Geometry check sheet. Reference: the model listing, model coordinates, mm. A direction names the side the tool comes from. Round coordinates to 2 decimals unless told otherwise and drop trailing zeros. Order: outer loops, then holes, each group sorted by start corner. A loop starts at its lowest first (then second) coordinate and runs counter-clockwise, first axis right, second up.
(1) Gauge pin test, flat ends, axial feed: P1, Ø1, axis at x = 761.5, y = 280.5, coming from the +Z side; P2, Ø12, axis at x = 488.5, y = 11.5, coming from the +Z side; P3, Ø2, axis at x = 1047, y = 98, coming from the +Z side. Record the tip position at first contact, or that the pin passes through.
(2) Thickness scan on L1, parallel to X at y = -38, z = -235; L2, parallel to Y at x = 744.5, z = -304; L3, parallel to Z at x = 1134.5, y = 121. Record the ranges inside material, lowest first.
(3) Cross-section at A-A on x = 1303.5. Enter the section's corners in (y, z), and give its area (3 significant figures).
(4) Cross-section at C-C on x = 779. Enter the section's corners in (y, z), and give its area (3 significant figures).
(5) Cross-section at D-D on x = 186. Enter the section's corners in (y, z).
(6) Set-up check for faces 1 (the face through (611.188, 123, -384)), 2 (the face through (759.89, 150.37, -368.76)), 3 (the face through (1068.911, 284.287, -296.554)), 4 (the face through (455.09, 144.39, -330.81)): record each of +Z, -Z, +X, -X, +Y, -Y from which the full face is reachable in a straight line by a thin tool's end or side.
(7) Cross-section at B-B on y = -107. Enter the section's corners in (x, z).
from build123d import *

# Parameters (mm, degrees)
F1_DEPTH  = 1524
F4_DEPTH  = 304.8
F7_DEPTH  = 304.8
F10_DEPTH = 304.8
F14_DEPTH = 1.5875
F16_DEPTH = 1.5875
F18_DEPTH = 1.5875
F20_DEPTH = 1.5875
F22_DEPTH = 1.5875
F24_DEPTH = 304.8
F26_DEPTH = 1.5875


with BuildPart() as f1:
    # F0 (on Right) → F1 (new body)
    with BuildSketch(Plane.YZ):
        with BuildLine():
            ThreePointArc((0, -347.4403916943), (-25.4, -372.8403916943), (0, -398.2403916943))
            ThreePointArc((0, -398.2403916943), (152.4, -367.9261469057), (281.5984815094, -281.5984815094))
            ThreePointArc((281.5984815094, -281.5984815094), (144.5967339925, -330.7608902035), (0, -347.4403916943))
        make_face()
    extrude(amount=F1_DEPTH)

    # F3 (on 3pt) → F4 (join)
    with BuildSketch(Plane.YZ.offset(1524)):
        Polygon((302.0386043773, -306.5287324379), (281.5984815094, -281.5984815094), (263.6379692673, -263.6379692673), (261.392905237, -265.8830332976), align=None)
    extrude(amount=-F4_DEPTH)

    # F6 (on offset) → F7 (join)
    with BuildSketch(Plane.YZ.offset(1219.2)):
        Polygon((286.9017213141, -311.0970612814), (281.5984815094, -281.5984815094), (274.4811571478, -257.216035079), (271.433351344, -258.1057006243), align=None)
    extrude(amount=-F7_DEPTH)

    # F9 (on offset) → F10 (join)
    with BuildSketch(Plane.YZ.offset(914.4)):
        Polygon((278.4234815094, -284.1384815094), (281.5984815094, -281.5984815094), (281.5984815094, -256.1984815094), (278.4234815094, -256.1984815094), align=None)
    extrude(amount=-F10_DEPTH)

    # F13 (on face) → F14 (join, symmetric)
    with BuildSketch(Plane(origin=(0, 0, 0), x_dir=(0, -1, 0), z_dir=(-1, 0, 0))):
        with BuildLine():
            ThreePointArc((0, -550.6403916943), (177.8, -372.8403916943), (0, -195.0403916943))
            ThreePointArc((0, -195.0403916943), (-109.8991760494, -182.3633178757), (-214.0258651779, -144.9979634939))
            ThreePointArc((-214.0258651779, -144.9979634939), (-405.4217806891, -192.7528255646), (-389.3615549623, -389.3615549623))
            ThreePointArc((-389.3615549623, -389.3615549623), (-210.7209550924, -508.7253876604), (0, -550.6403916943))
        make_face()
    extrude(amount=F14_DEPTH, both=True)

    # F15 (on offset) → F16 (join, symmetric)
    with BuildSketch(Plane.YZ.offset(609.6)):
        with BuildLine():
            ThreePointArc((211.9278055472, -146.0295007467), (108.760588215, -182.6280830102), (0, -195.0403916943))
            ThreePointArc((0, -195.0403916943), (-177.8, -372.8403916943), (0, -550.6403916943))
            ThreePointArc((0, -550.6403916943), (210.7209550924, -508.7253876604), (389.3615549623, -389.3615549623))
            ThreePointArc((389.3615549623, -389.3615549623), (402.6332177904, -193.3271563276), (211.9278055472, -146.0295007467))
        make_face()
    extrude(amount=F16_DEPTH, both=True)

    # F17 (on offset) → F18 (join, symmetric)
    with BuildSketch(Plane.YZ.offset(914.4)):
        with BuildLine():
            ThreePointArc((211.9278055472, -146.0295007467), (108.760588215, -182.6280830102), (0, -195.0403916943))
            ThreePointArc((0, -195.0403916943), (-177.8, -372.8403916943), (0, -550.6403916943))
            ThreePointArc((0, -550.6403916943), (210.7209550924, -508.7253876604), (389.3615549623, -389.3615549623))
            ThreePointArc((389.3615549623, -389.3615549623), (402.6332177904, -193.3271563276), (211.9278055472, -146.0295007467))
        make_face()
    extrude(amount=F18_DEPTH, both=True)

    # F19 (on offset) → F20 (join, symmetric)
    with BuildSketch(Plane.YZ.offset(1219.2)):
        with BuildLine():
            ThreePointArc((211.9278055472, -146.0295007467), (108.760588215, -182.6280830102), (0, -195.0403916943))
            ThreePointArc((0, -195.0403916943), (-177.8, -372.8403916943), (0, -550.6403916943))
            ThreePointArc((0, -550.6403916943), (210.7209550924, -508.7253876604), (389.3615549623, -389.3615549623))
            ThreePointArc((389.3615549623, -389.3615549623), (402.6332177904, -193.3271563276), (211.9278055472, -146.0295007467))
        make_face()
    extrude(amount=F20_DEPTH, both=True)

    # F21 (on 3pt) → F22 (join, symmetric)
    with BuildSketch(Plane.YZ.offset(1524)):
        with BuildLine():
            ThreePointArc((211.9278055472, -146.0295007467), (108.760588215, -182.6280830102), (0, -195.0403916943))
            ThreePointArc((0, -195.0403916943), (-177.8, -372.8403916943), (0, -550.6403916943))
            ThreePointArc((0, -550.6403916943), (210.7209550924, -508.7253876604), (389.3615549623, -389.3615549623))
            ThreePointArc((389.3615549623, -389.3615549623), (402.6332177904, -193.3271563276), (211.9278055472, -146.0295007467))
        make_face()
    extrude(amount=F22_DEPTH, both=True)

    # F23 (on offset) → F24 (join)
    with BuildSketch(Plane.YZ.offset(609.6)):
        Polygon((277.4514655912, -283.945135522), (281.5984815094, -281.5984815094), (291.3186406915, -258.1319413837), (288.1436406915, -258.1319413837), align=None)
    extrude(amount=-F24_DEPTH)

    # F25 (on offset) → F26 (join, symmetric)
    with BuildSketch(Plane.YZ.offset(304.8)):
        with BuildLine():
            ThreePointArc((211.1335691615, -146.4167113639), (108.3301046752, -182.7274300654), (0, -195.0403916943))
            ThreePointArc((0, -195.0403916943), (-177.8, -372.8403916943), (0, -550.6403916943))
            ThreePointArc((0, -550.6403916943), (210.7209550924, -508.7253876604), (389.3615549623, -389.3615549623))
            ThreePointArc((389.3615549623, -389.3615549623), (401.5869061697, -193.5450684149), (211.1335691615, -146.4167113639))
        make_face()
    extrude(amount=F26_DEPTH, both=True)


solid = f1.part
Found:
1. P1: stops at z = -256.2
1. P2: stops at z = -347.2
1. P3: stops at z = -339.68
2. L1: x = -1.59 to 1.59, 303.21 to 306.39, 608.01 to 611.19, 912.81 to 915.99, 1217.61 to 1220.79, 1522.41 to 1525.59
2. L2: y = 230.85 to 257.25
2. L3: z = -379.41 to -335.81
3. outline: (0, -398.24) arc R398.24 ccw to (279.34, -283.83) - (302.04, -306.53) - (281.6, -281.6) - (263.64, -263.64) - (261.39, -265.88) - (278.59, -283.08) arc R635.1 cw to (0, -347.44) arc R25.4 ccw to start
3. area: 11,300 mm2
4. outline: (0, -398.24) arc R398.24 ccw to (281.6, -281.6) - (281.6, -256.2) - (278.42, -256.2) - (278.42, -283.16) arc R635.1 cw to (0, -347.44) arc R25.4 ccw to start
4. area: 11,200 mm2
5. outline: (0, -398.24) arc R398.24 ccw to (281.6, -281.6) arc R635.1 cw to (0, -347.44) arc R25.4 ccw to start
6. face 1: none
6. face 2: -Z, +Y
6. face 3: +Z, +Y
6. face 4: +Z, -Y
7. outline: (-1.59, -514.84) - (1.59, -514.84) - (1.59, -230.84) - (-1.59, -230.84) - close; (303.21, -514.84) - (306.39, -514.84) - (306.39, -230.84) - (303.21, -230.84) - close; (608.01, -514.84) - (611.19, -514.84) - (611.19, -230.84) - (608.01, -230.84) - close; (912.81, -514.84) - (915.99, -514.84) - (915.99, -230.84) - (912.81, -230.84) - close; (1217.61, -514.84) - (1220.79, -514.84) - (1220.79, -230.84) - (1217.61, -230.84) - close; (1522.41, -514.84) - (1525.59, -514.84) - (1525.59, -230.84) - (1522.41, -230.84) - close
